Geometry check sheet. Reference: drawing and pictorial views, mm from the part's lowest x, y, z. Round coordinates to 2 decimals unless told otherwise and drop trailing zeros. Write each loop counter-clockwise with the first axis right and the second up, starting at its lowest first coordinate (ties: lowest second). Pieces come first, ordered by that corner, then holes. Notation, with made-up numbers: M 77.5,36 L 103.5,36 A23 ccw 103.5,73 Z; hole C 30,-36.5 d7. An arc over 180 degrees is marked long. Use a Markdown table: item, result. Add a question column.
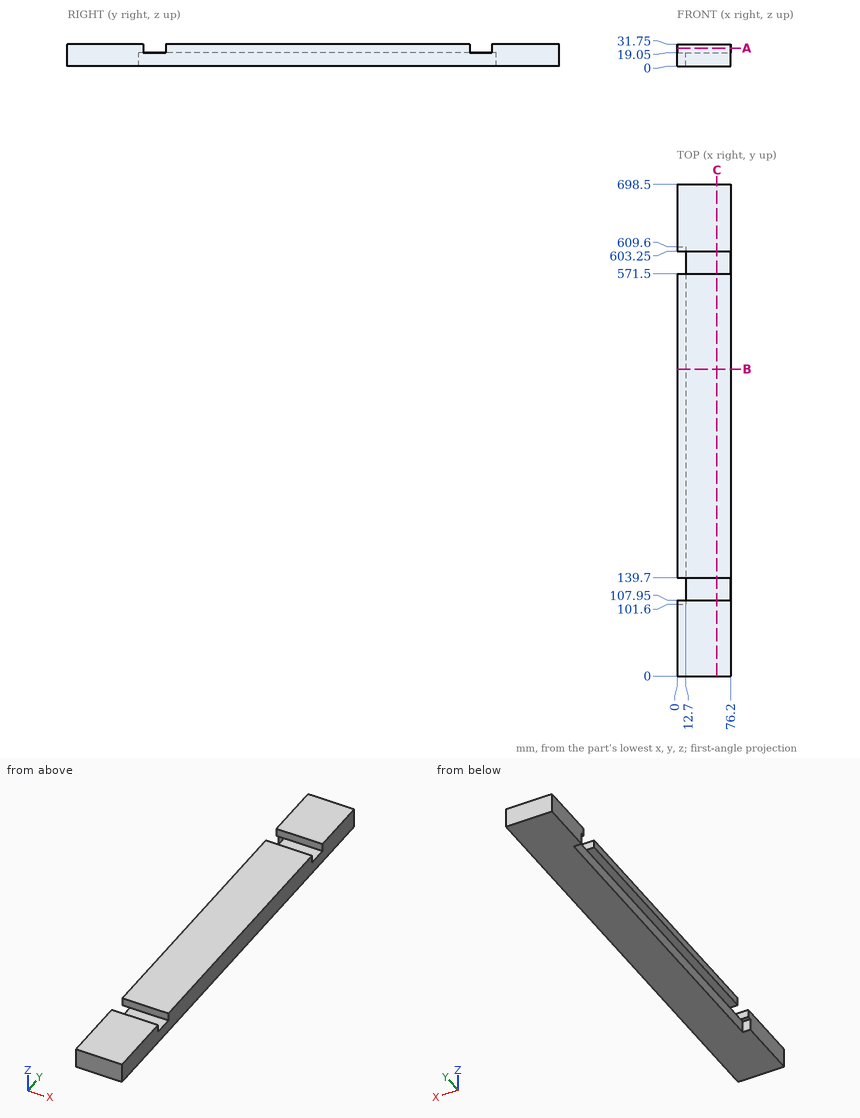
1. Cross-section at C-C on x = 56.5. Enter the section's corners in (y, z).
2. Depth check by flat-ended pin: pin 1 Ø5 at (x, y) = (27.5, 574.5) entering from +Z; pin 2 Ø3 at (x, y) = (4.5, 104) entering from -Z; pin 3 Ø4 at (x, z) = (32, 22.5) entering from -Y; pin 4 Ø1.5 at (y, z) = (385, 6.5) entering from -X. Enter the tip coordinate at first touch or a pass-through.
3. Scan lines: line 1 along Y through (x, z) = (26, 24); line 2 along Y through (x, z) = (8.5, 18); line 3 along X through (y, z) = (147.5, 15). Record each from-to range of solid material in increasing order. Write a range as from..to.
4. Cross-section at A-A on z = 26. Enter the section's corners in (x, y).
5. Cross-section at B-B on y = 436. Enter the section's corners in (x, z), plus the area to 3 significant figures.
Answer:
| question | item | result |
|---|---|---|
| 1 | outline | M 0,0 L 698.5,0 L 698.5,31.75 L 603.25,31.75 L 603.25,19.05 L 571.5,19.05 L 571.5,31.75 L 139.7,31.75 L 139.7,19.05 L 107.95,19.05 L 107.95,31.75 L 0,31.75 Z |
| 2 | pin 1 | stops at z = 19.05 |
| 2 | pin 2 | stops at z = 19.05 |
| 2 | pin 3 | stops at y = 0 |
| 2 | pin 4 | stops at x = 12.7 |
| 3 | line 1 | y = 0..107.95, 139.7..571.5, 603.25..698.5 |
| 3 | line 2 | y = 0..101.6, 609.6..698.5 |
| 3 | line 3 | x = 12.7..76.2 |
| 4 | outline | M 0,0 L 76.2,0 L 76.2,107.95 L 0,107.95 Z; M 0,139.7 L 76.2,139.7 L 76.2,571.5 L 0,571.5 Z; M 0,603.25 L 76.2,603.25 L 76.2,698.5 L 0,698.5 Z |
| 5 | outline | M 0,19.05 L 12.7,19.05 L 12.7,0 L 76.2,0 L 76.2,31.75 L 0,31.75 Z |
| 5 | area | 2,180 mm^2 |
